Read the model definition and answer for the solid it produces. Units are mm, in the model's axes. Give positions to 0.01 mm unless a question says otherwise; leave off trailing zeros. Order: outer loops, then holes, each group sorted by start corner. A loop starts at its lowest first (then second) coordinate and runs counter-clockwise, first axis right, second up.
Item 1: A cutting plane is placed at A-A (z = 3.45). State how many separate pieces and enclosed holes the cut face has, plus the area to 3 significant figures.
Item 2: Find the intervals of material crossed by line 1 along Y through (x, z) = (351.5, 5.85); line 2 along X through (y, z) = (-7.5, 4.6); line 3 along X through (y, z) = (-45, 0.85), in increasing order.
Item 3: Given pin 1 Ø0.9 at (y, z) = (-42, 2) entering from -X; pin 2 Ø1.8 at (y, z) = (-2, 4.5) entering from -X; pin 3 Ø1.8 at (x, z) = (377.5, 3) entering from +Y; pin 4 Ø6 at (x, y) = (247.5, -58.5) entering from -Z, each flat-ended and moving along its own axis, determine where each tip first touches the part or whether it passes through.
Item 4: A cutting plane is placed at B-B (y = -32). Write down the section's boundary in (x, z).
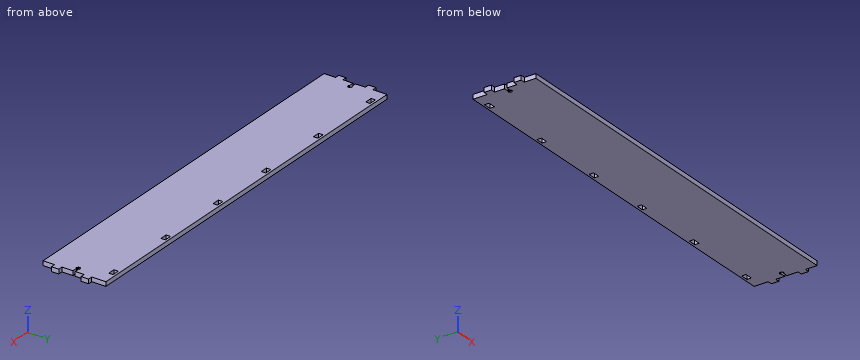
from build123d import *

# Parameters (mm, degrees)
SKETCH_1_W      = 10
SKETCH_1_H      = 6
EXTRUDE_1_DEPTH = 6


with BuildPart() as part:
    # Эскиз1 → Бобышка-Вытянуть1 (new body)
    with BuildSketch(Plane.XY):
        Polygon((-164.373633731, 3), (373.626366269, 3), (373.626366269, -16.168156269), (379.626366269, -16.168156269), (379.626366269, -26.168156269), (373.626366269, -26.168156269), (373.626366269, -38.45), (366.754885836, -38.45), (366.754885836, -37.25), (364.554885836, -37.25), (364.554885836, -38.45), (363.054885836, -38.45), (363.054885836, -41.55), (364.554885836, -41.55), (364.554885836, -42.75), (366.754885836, -42.75), (366.754885836, -41.55), (373.626366269, -41.55), (373.626366269, -56.331843731), (379.626366269, -56.331843731), (379.626366269, -66.331843731), (373.626366269, -66.331843731), (373.626366269, -82), (-164.373633731, -82), (-164.373633731, -66.331843731), (-170.373633731, -66.331843731), (-170.373633731, -56.331843731), (-164.373633731, -56.331843731), (-164.302153297, -42.8), (-164.230672864, -42.8), (-157.430672864, -42.8), (-157.430672864, -44), (-155.230672864, -44), (-155.230672864, -42.8), (-153.730672864, -42.8), (-153.730672864, -39.7), (-155.230672864, -39.7), (-155.230672864, -38.5), (-157.430672864, -38.5), (-157.430672864, -39.7), (-164.230672864, -39.7), (-164.302153297, -39.7), (-164.373633731, -26.168156269), (-170.373633731, -26.168156269), (-170.373633731, -16.168156269), (-164.373633731, -16.168156269), align=None)
        with Locations((-141.373633731, -3)):
            Rectangle(SKETCH_1_W, SKETCH_1_H, mode=Mode.SUBTRACT)
        with Locations((-41.373633731, -3)):
            Rectangle(SKETCH_1_W, SKETCH_1_H, mode=Mode.SUBTRACT)
        with Locations((58.626366269, -3)):
            Rectangle(SKETCH_1_W, SKETCH_1_H, mode=Mode.SUBTRACT)
        with Locations((150.626366269, -3)):
            Rectangle(SKETCH_1_W, SKETCH_1_H, mode=Mode.SUBTRACT)
        with Locations((250.626366269, -3)):
            Rectangle(SKETCH_1_W, SKETCH_1_H, mode=Mode.SUBTRACT)
        with Locations((350.626366269, -3)):
            Rectangle(SKETCH_1_W, SKETCH_1_H, mode=Mode.SUBTRACT)
    extrude(amount=EXTRUDE_1_DEPTH)


solid = part.part
Response values:
1. separate pieces: 1
1. enclosed holes: 6
1. area: 45,500 mm2
2. line 1: y = -82 to -6, 0 to 3
2. line 2: x = -164.37 to 373.63
2. line 3: x = -164.31 to 373.63
3. pin 1: stops at x = -153.73
3. pin 2: stops at x = -164.37
3. pin 3: stops at y = -16.17
3. pin 4: stops at z = 0
4. outline: (-164.34, 0) - (373.63, 0) - (373.63, 6) - (-164.34, 6) - close
